from build123d import *

# Parameters (mm, degrees)
SKETCH_W     = 15
SKETCH_H     = 33
PAD_DEPTH    = 6
SKETCH001_R  = 5.1
PAD001_DEPTH = 3
SKETCH002_R  = 4.1
POCKET_DEPTH = 9.001
FILLET_R     = 4


with BuildPart() as part:
    # Sketch → Pad (new body)
    with BuildSketch(Plane.XY):
        with Locations((7.5, 16.5)):
            Rectangle(SKETCH_W, SKETCH_H)
    extrude(amount=PAD_DEPTH)

    # Sketch001 → Pad001 (new body)
    with BuildSketch(Plane.XY.offset(6)):
        with Locations((7.5, 28)):
            Circle(SKETCH001_R)
    extrude(amount=PAD001_DEPTH)

    # Sketch002 → Pocket (cut, through all)
    with BuildSketch(Plane.XY.offset(9)):
        with Locations((7.5, 28)):
            Circle(SKETCH002_R)
    extrude(amount=-POCKET_DEPTH, mode=Mode.SUBTRACT)

    # Fillet
    fillet_edges = [part.edges().sort_by_distance(p)[0] for p in [
        (0, 0, 3),
        (15, 0, 3),
    ]]
    fillet(fillet_edges, radius=FILLET_R)


solid = part.part
Can you work these out from the model? Positions are in its coordinate system, mm. A direction names the side the tool comes from. Give positions to 0.01 mm unless a question says otherwise; leave off trailing zeros. Write each loop counter-clockwise with the first axis right and the second up, starting at its lowest first coordinate (ties: lowest second). Pieces come first, ordered by that corner, then holes. Notation, with made-up numbers: M -9,10.25 L 41,10.25 A24 cw 41,22.25 Z; hole C -13.5,-12.75 d1. An arc over 180 degrees is marked long. Answer in a Markdown table with one row per item. Add a question column.
Item 1: Please list where these lines run through material, in increasing order: L1, parallel to Y at x = 7.5, z = 4.75; L2, parallel to Z at x = 14, y = 22; L3, parallel to Y at x = 8.5, z = 2.
Item 2: Imagine slicing it at A-A, the plane y = 28. Write out the boundary of the cut face in (x, z), plus the area to 3 significant figures.
Item 3: Imagine slicing it at D-D, the plane z = 6.75. Write out the boundary of the cut face in (x, y).
Item 4: Imagine slicing it at C-C, the plane z = 1.25. Write out the boundary of the cut face in (x, y).
Item 5: We'd pull the mould along X, two halves only. Please class faces 1 (the cylindrical face through (6.6, 24, 4.6)), 2 (the flat face through (0, 18, 3)), 3 (the flat face through (12, 28, 9)): released by +X, released by -X, zero draft, split by the parting line, or undercut.
Item 6: On a 3-axis mill with a long thin cutter (end or side, diameter ignored), from which of +Z, -Z, +X, -X, +Y, -Y can I reach the whole of each face in a straight line? I mean faces 4 (the cylindrical face through (6.394, 23.021, 7.479)), 5 (the cylindrical face through (1.141, 1.203, 3.042)). Say none if no direction works.
Item 7: For pin 1 Ø4 at (x, z) = (1.5, 2) entering from -Y; pin 2 Ø2 at (x, y) = (12, 5.5) entering from +Z; pin 3 Ø3 at (x, z) = (10.5, 4.5) entering from +Y, each with a flat end and sliding along its axis, tell me the tip position at first contact or that it passes through.
Item 8: Imagine slicing it at B-B, the plane x = 7.5. Write out the boundary of the cut face in (y, z), plus the area to 3 significant figures.
Evaluation:
| question | item | result |
|---|---|---|
| 1 | L1 | y = 0 to 23.9, 32.1 to 33 |
| 1 | L2 | z = 0 to 6 |
| 1 | L3 | y = 0 to 24.02, 31.98 to 33 |
| 2 | outline | M 0,0 L 3.4,0 L 3.4,9 L 2.4,9 L 2.4,6 L 0,6 Z; M 11.6,0 L 15,0 L 15,6 L 12.6,6 L 12.6,9 L 11.6,9 Z |
| 2 | area | 46.8 mm² |
| 3 | outline | C 7.5,28 d10.2; hole C 7.5,28 d8.2 |
| 4 | outline | M 0,4 A4 ccw 4,0 L 11,0 A4 ccw 15,4 L 15,33 L 0,33 Z; hole C 7.5,28 d8.2 |
| 5 | face 1 | undercut |
| 5 | face 2 | released by -X |
| 5 | face 3 | zero draft |
| 6 | face 4 | +Z |
| 6 | face 5 | +Z, -Z, -X, -Y |
| 7 | pin 1 | stops at y = 0.03 |
| 7 | pin 2 | stops at z = 6 |
| 7 | pin 3 | stops at y = 33 |
| 8 | outline | M 0,0 L 23.9,0 L 23.9,9 L 22.9,9 L 22.9,6 L 0,6 Z; M 32.1,0 L 33,0 L 33,6 L 33.1,6 L 33.1,9 L 32.1,9 Z |
| 8 | area | 155 mm² |
